Design review of the part shown in the three views and the two pictorial views. Dimensions are in mm from the part's minimum x, y and z. Give positions to 0.01 mm unless a question says otherwise; leave off trailing zeros. Write each loop counter-clockwise with the first axis right and the second up, starting at its lowest first coordinate (ties: lowest second). Pieces come first, ordered by that corner, then holes.
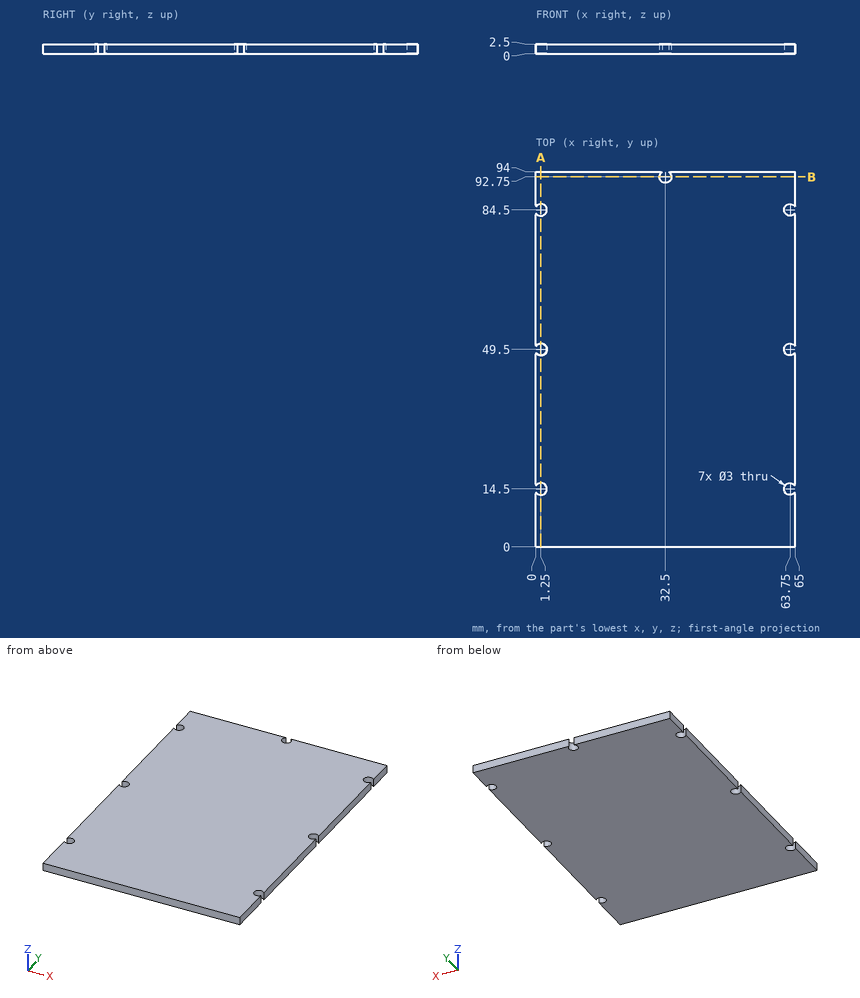
(1) To check wall thickness, follow L1, parallel to Y at x = 1.25, z = 1.15; L2, parallel to X at y = 92.75, z = 0.9; L3, parallel to X at y = 49.5, z = 1.7. State the ranges of each line that lie inside material, in increasing order.
Resolved:
L1: y = 0 to 13, 16 to 48, 51 to 83, 86 to 94
L2: x = 0 to 31, 34 to 65
L3: x = 2.75 to 62.25
(2) Consider section A-A, the plane x = 1.25. Give the boundary of the cut face in (y, z), then the cut area to 4 significant figures.
Resolved:
outline: (0, 0) - (13, 0) - (13, 2.5) - (0, 2.5) - close; (16, 0) - (48, 0) - (48, 2.5) - (16, 2.5) - close; (51, 0) - (83, 0) - (83, 2.5) - (51, 2.5) - close; (86, 0) - (94, 0) - (94, 2.5) - (86, 2.5) - close
area: 212.5 mm2
(3) Consider section B-B, the plane y = 92.75. Give the boundary of the cut face in (x, z).
Resolved:
outline: (0, 0) - (31, 0) - (31, 2.5) - (0, 2.5) - close; (34, 0) - (65, 0) - (65, 2.5) - (34, 2.5) - close
